Could you check a few things on this model? Use its own coordinates, in mm. A direction names the side the tool comes from. Coordinates: 2 decimals unless noted, no trailing zeros. Write each loop counter-clockwise with the first axis right and the second up, starting at its lowest first coordinate (ties: lowest second). Pieces come first, ordered by that corner, then holes. Notation, with made-up numbers: (-33.5, -22) - (24.5, -22) arc R20 ccw to (24.5, 9) - close; hole circle Ø3 at (-8.75, -8). An arc over 180 degrees is marked (long way). Answer as a JSON object with one key per item and string values. Group by question number.
1) Please list where these lines run through material, in increasing order: line 1 along X through (y, z) = (0, 2.5); line 2 along Y through (x, z) = (-24.5, 4.5); line 3 along X through (y, z) = (22.5, 2.5).
2) If we section it at B-B (x = 0): Write out the boundary of the cut face in (y, z).
3) On a 3-axis mill with a long thin cutter (end or side, diameter ignored), from which of +Z, -Z, +X, -X, +Y, -Y can I reach the whole of each face in a straight line? I mean faces 4 (the flat face through (-0.3, 47.2, 10)), 5 (the flat face through (-11.651, -50, 5)). Say none if no direction works.
4) If we section it at C-C (z = 4.25): Write out the boundary of the cut face in (x, y), plus the area to 3 significant figures.
5) We'd pull the mould along X, two halves only. Please class faces 1 (the conical face through (1.826, 45.088, 8.125)), 2 (the flat face through (17, 43, 0)), 3 (the cylindrical face through (2.36, 57.45, 4.93)): released by +X, released by -X, zero draft, split by the parting line, or undercut.
6) If we section it at A-A (y = 0): Write out the boundary of the cut face in (x, z).
7) Will these pins go through, and if not, where does the flat tip stop? pin 1 Ø5 at (x, z) = (41, 5.5) entering from +Y; pin 2 Ø3 at (y, z) = (-51.5, 4) entering from -X; pin 3 Ø1 at (x, y) = (43, 4.5) entering from +Z; pin 4 Ø5 at (y, z) = (-8.5, 3) entering from +X.
```python
from build123d import *

# Parameters (mm, degrees)
SKETCH1_R           = 57.5
SKETCH1_R_2         = 45
BOSS_EXTRUDE1_DEPTH = 10
CUT_EXTRUDE2_DEPTH  = 10


with BuildPart() as part:
    # Sketch1 → Boss-Extrude1 (new body)
    with BuildSketch(Plane(origin=(0, 0, 0), x_dir=(0, 1, 0), z_dir=(0, 0, 1))):
        with Locations(Location((0, 0, 0), (0, 0, 270))):
            Circle(SKETCH1_R)
        with Locations(Location((0, 0, 0), (0, 0, 270))):
            Circle(SKETCH1_R_2, mode=Mode.SUBTRACT)
    extrude(amount=BOSS_EXTRUDE1_DEPTH)

    # Sketch2 → Cut-Extrude2 (cut)
    with BuildSketch(Plane(origin=(0, 0, 0), x_dir=(1, 0, 0), z_dir=(0, 0, -1))):
        with BuildLine():
            Line((11.650511373, 56.659857386), (11.650511373, 43.46568284))
            add(Edge.make_bspline(
                [(11.650511373, 43.46568284), (-0.679246558, 46.406413024), (-11.650511373, 43.46568284)],
                knots=[0, 0, 0, 0.575547458, 0.575547458, 0.575547458], degree=2))
            Line((-11.650511373, 43.46568284), (-11.650511373, 56.659857386))
            ThreePointArc((-11.650511373, 56.659857386), (0, 57.845257837), (11.650511373, 56.659857386))
        make_face()
    extrude(amount=-CUT_EXTRUDE2_DEPTH, mode=Mode.SUBTRACT)

    # Chamfer1: read off the stored shape, not the designer's step
    # Chamfer1 outline → Chamfer1 (revolve, cut)
    with BuildSketch(Plane.XZ):
        Polygon((45, 10.000000111), (45, 8), (47.000000111, 10.000000111), align=None)
    revolve(axis=Axis((0, 0, 0), (0, 0, 1)), mode=Mode.SUBTRACT)


solid = part.part
```
Here are the results:
{
 "1": {"line 1": "x = -57.5 to -45, 45 to 57.5", "line 2": "y = -52.02 to -37.75, 37.75 to 52.02", "line 3": "x = -52.92 to -38.97, 38.97 to 52.92"},
 "2": {"outline": "(45, 0) - (57.5, 0) - (57.5, 10) - (47, 10) - (45, 8) - close"},
 "3": {"face 4": "+Z, +X, -X, +Y, -Y", "face 5": "+Z, -Z, -Y"},
 "4": {"outline": "(-11.65, -56.31) - (-11.65, -43.47) arc R45 cw (long way) to (11.65, -43.47) - (11.65, -56.31) arc R57.5 ccw (long way) to start", "area": "3,730 mm²"},
 "5": {"face 1": "undercut", "face 2": "zero draft", "face 3": "split by the parting line"},
 "6": {"outline": "(-57.5, 0) - (-45, 0) - (-45, 8) - (-47, 10) - (-57.5, 10) - close; (45, 0) - (57.5, 0) - (57.5, 10) - (47, 10) - (45, 8) - close"},
 "7": {"pin 1": "stops at y = 42.71", "pin 2": "stops at x = -28.39", "pin 3": "passes through", "pin 4": "stops at x = 57.19"}
}
